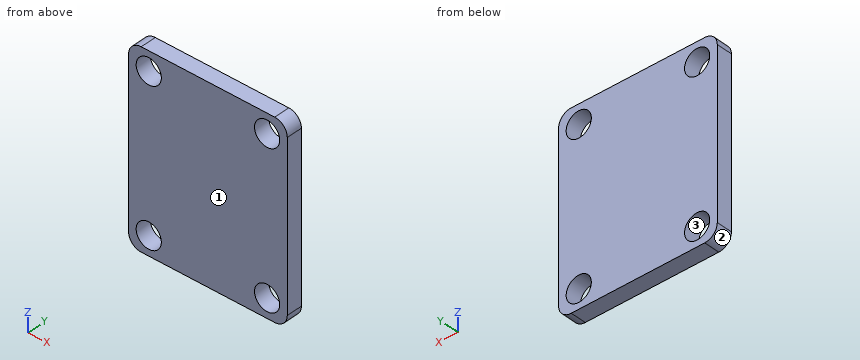
```python
from build123d import *

# Parameters (mm, degrees)
SKETCH3_W           = 32.004
SKETCH3_H           = 38.1
BOSS_EXTRUDE1_DEPTH = 3.175
SKETCH4_R           = 2.54
CUT_EXTRUDE1_DEPTH  = 26.080811969
FILLET1_R           = 2.54


with BuildPart() as part:
    # Sketch3 → Boss-Extrude1 (new body)
    with BuildSketch(Plane(origin=(0, 0, 0), x_dir=(1, 0, 0), z_dir=(0, 1, 0))):
        Rectangle(SKETCH3_W, SKETCH3_H)
    extrude(amount=-BOSS_EXTRUDE1_DEPTH)

    # Sketch4 → Cut-Extrude1 (cut, through all)
    with BuildSketch(Plane(origin=(0, 0, 0), x_dir=(1, 0, 0), z_dir=(0, 1, 0))):
        with Locations(Location((11.938, 15.24, 0), (0, 0, 270))):
            Circle(SKETCH4_R)
        with Locations(Location((-11.938, 15.24, 0), (0, 0, 270))):
            Circle(SKETCH4_R)
        with Locations(Location((-11.938, -15.24, 0), (0, 0, 270))):
            Circle(SKETCH4_R)
        with Locations(Location((11.938, -15.24, 0), (0, 0, 270))):
            Circle(SKETCH4_R)
    extrude(amount=-CUT_EXTRUDE1_DEPTH, mode=Mode.SUBTRACT)

    # Fillet1
    fillet1_edges = [part.edges().sort_by_distance(p)[0] for p in [
        (-16.002, -1.5875, -19.05),
        (16.002, -1.5875, -19.05),
        (16.002, -1.5875, 19.05),
        (-16.002, -1.5875, 19.05),
    ]]
    fillet(fillet1_edges, radius=FILLET1_R)


solid = part.part
```
The model under review builds one solid part; all positions refer to its coordinate system, in mm. Face numbers are marked on the shaded views. Round coordinates to 2 decimals unless told otherwise and drop trailing zeros. Loops run counter-clockwise (first coordinate to the right, second up) from the corner with the lowest first, then second, coordinate; pieces in that order, holes last.
1) Consider section A-A on z = -15.24. State the section outline as (x, y) points (3 decimals).
Values follow:
outline: (-16.002, -3.175) - (-14.478, -3.175) - (-14.478, 0) - (-16.002, 0) - close; (-9.398, -3.175) - (9.398, -3.175) - (9.398, 0) - (-9.398, 0) - close; (14.478, -3.175) - (16.002, -3.175) - (16.002, 0) - (14.478, 0) - close
2) Consider section B-B on y = -1.8. State the section outline as (x, z) points.
Values follow:
outline: (-16, -16.51) arc R2.54 ccw to (-13.46, -19.05) - (13.46, -19.05) arc R2.54 ccw to (16, -16.51) - (16, 16.51) arc R2.54 ccw to (13.46, 19.05) - (-13.46, 19.05) arc R2.54 ccw to (-16, 16.51) - close; hole circle Ø5.08 at (-11.94, -15.24); hole circle Ø5.08 at (-11.94, 15.24); hole circle Ø5.08 at (11.94, -15.24); hole circle Ø5.08 at (11.94, 15.24)
3) Clearance check with a flat-ended pin moving along its axis: P1, Ø3, axis at x = 11.938, z = 15.24, coming from the -Y side. State where the tip first meets the part, or that it passes through.
Values follow:
P1: passes through
4) Wall thickness on line 1 along X through (y, z) = (-1.1, -15.24); line 2 along Z through (x, y) = (-12, -2.4); line 3 along Z through (x, y) = (-11.5, -2.65): over which ranges is each line inside the solid? List them lowest first.
Values follow:
line 1: x = -16 to -14.48, -9.4 to 9.4, 14.48 to 16
line 2: z = -19.05 to -17.78, -12.7 to 12.7, 17.78 to 19.05
line 3: z = -19.05 to -17.74, -12.74 to 12.74, 17.74 to 19.05
5) The part is to be moulded in two halves that separate along Z. For the marked faces 1, 2 and 3, say which applies: pulls with the +Z half, pulls with the -Z half, needs draft (parallel to the pull), parting line crosses it, or undercut.
Values follow:
face 1: needs draft
face 2: pulls with the -Z half
face 3: undercut
